The model under review builds one solid part; all positions refer to its coordinate system, in mm. Coordinates: 2 decimals unless noted, no trailing zeros. Loops run counter-clockwise (first coordinate to the right, second up) from the corner with the lowest first, then second, coordinate; pieces in that order, holes last. Notation, with made-up numbers: M 26.25,89.5 L 78.25,89.5 A7 cw 78.25,97.5 Z; hole C -25.5,63 d7. An arc over 180 degrees is marked long. Use one line per item in the form item = value.
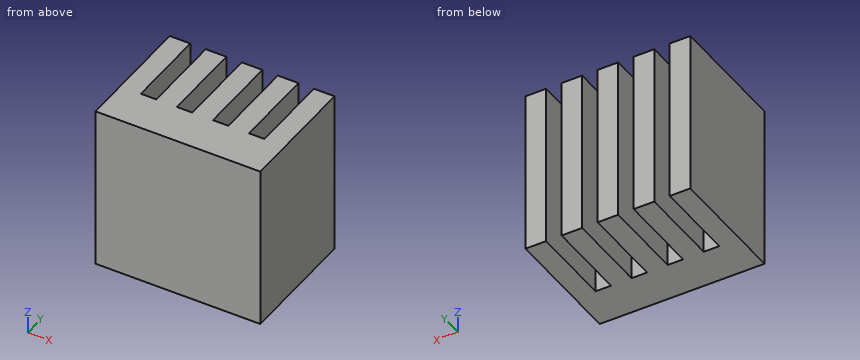
Autodesk Inventor part; units mm, degrees
ref_plane "YZ Plane" through (0, 0, 0) normal (1, 0, 0) x (0, 1, 0)
ref_plane "XZ Plane" through (0, 0, 0) normal (0, 1, 0) x (-1, 0, 0)
ref_plane "XY Plane" through (0, 0, 0) normal (0, 0, 1) x (1, 0, 0)
sketch "Sketch1" plane through (0, 0, 0) normal (0, 0, 1) x (1, 0, 0)
  line L0 (-4.5765, 3.9949) -> (3.4235, 3.9949)
  line L1 (3.4235, 3.9949) -> (3.4235, -2.0051)
  line L2 (3.4235, -2.0051) -> (-4.5765, -2.0051)
  line L3 (-4.5765, -2.0051) -> (-4.5765, 3.9949)
  line L4 (-4.5765, -0.0051) -> (3.4235, -0.0051)
  line L5 (-3.5765, 3.9949) -> (-2.8265, 3.9949)
  line L6 (-2.8265, 3.9949) -> (-2.8265, -0.0051)
  line L7 (-2.8265, -0.0051) -> (-3.5765, -0.0051)
  line L8 (-3.5765, -0.0051) -> (-3.5765, 3.9949)
  line L9 (-1.8265, 3.9949) -> (-1.0765, 3.9949)
  line L10 (-1.0765, 3.9949) -> (-1.0765, -0.0051)
  line L11 (-1.0765, -0.0051) -> (-1.8265, -0.0051)
  line L12 (-1.8265, -0.0051) -> (-1.8265, 3.9949)
  line L13 (1.6735, 3.9949) -> (2.4235, 3.9949)
  line L14 (2.4235, 3.9949) -> (2.4235, -0.0051)
  line L15 (2.4235, -0.0051) -> (1.6735, -0.0051)
  line L16 (1.6735, -0.0051) -> (1.6735, 3.9949)
  line L17 (-0.0765, 3.9949) -> (0.6735, 3.9949)
  line L18 (0.6735, 3.9949) -> (0.6735, -0.0051)
  line L19 (0.6735, -0.0051) -> (-0.0765, -0.0051)
  line L20 (-0.0765, -0.0051) -> (-0.0765, 3.9949)
  point P0 (0, 0)
  dimension "d0" = 6
  dimension "d1" = 8
  dimension "d2" = 2
  dimension "d3" = 1
  dimension "d4" = 1
  dimension "d5" = 1
  dimension "d6" = 1
  dimension "d7" = 1
  dimension "d8" = 0.75
  dimension "d9" = 0.75
  dimension "d10" = 0.75
extrude "Extrusion1" add sketch "Sketch1" along normal blind 8 contours L0 L8 L4 L3 | L4 L1 L2 L3 | L0 L12 L4 L6 | L0 L20 L4 L10 | L4 L14 L0 L1 | L0 L16 L4 L18
properties part number "SmallHeatsink"
1. Insertion check: P1, Ø0.8, axis at x = -3.5, z = 3.5, coming from the +Y side. The pin has a flat end and moves straight along its axis. Give the tip position at first contact, or say it passes through.
Response values:
P1 = 3.99
2. Add section C-C (x = -1.25). State the section outline as (y, z) points, then the cut area to 3 significant figures.
Response values:
outline = M -2.01,0 L -0.01,0 L -0.01,8 L -2.01,8 Z
area = 16.0 mm^2
3. Add section B-B (z = 5.25). State the section outline as (x, y) points, then the cut area to 3 significant figures.
Response values:
outline = M -4.58,-2.01 L 3.42,-2.01 L 3.42,3.99 L 2.42,3.99 L 2.42,-0.01 L 1.67,-0.01 L 1.67,3.99 L 0.67,3.99 L 0.67,-0.01 L -0.08,-0.01 L -0.08,3.99 L -1.08,3.99 L -1.08,-0.01 L -1.83,-0.01 L -1.83,3.99 L -2.83,3.99 L -2.83,-0.01 L -3.58,-0.01 L -3.58,3.99 L -4.58,3.99 Z
area = 36.0 mm^2
4. Add section A-A (y = 1.35). State the section outline as (x, z) points.
Response values:
outline = M -4.58,0 L -3.58,0 L -3.58,8 L -4.58,8 Z; M -2.83,0 L -1.83,0 L -1.83,8 L -2.83,8 Z; M -1.08,0 L -0.08,0 L -0.08,8 L -1.08,8 Z; M 0.67,0 L 1.67,0 L 1.67,8 L 0.67,8 Z; M 2.42,0 L 3.42,0 L 3.42,8 L 2.42,8 Z
5. Wall thickness on line 1 along X through (y, z) = (0.75, 7); line 2 along Y through (x, z) = (0, 0.75): over which ranges is each line inside the solid? List them lowest first. Write a range as from..to.
Response values:
line_1 = -4.58..-3.58, -2.83..-1.83, -1.08..-0.08, 0.67..1.67, 2.42..3.42
line_2 = -2.01..-0.01
